For this review, take the finished solid that the model builds, in its own axes (mm). Round coordinates to 2 decimals unless told otherwise and drop trailing zeros. Write each loop counter-clockwise with the first axis right and the second up, starting at its lowest first coordinate (ties: lowest second). Pieces come first, ordered by that corner, then holes. Notation, with made-up numbers: (-31, 79) -> (-24, 79) arc R18 ccw to (-24, 83) -> close; hole circle Ø10 at (22, 85). An arc over 180 degrees is marked (long way). Write each question's results on one line, items separated by ' | '. Start each with the question number.
Item 1: Add section D-D (z = 2.2). State the section outline as (x, y) points.
Item 2: Add section B-B (y = 45.5). State the section outline as (x, z) points.
Item 3: Add section C-C (x = -1). State the section outline as (y, z) points, plus the area to 3 significant figures.
Item 4: To check wall thickness, follow line 1 along Z through (x, y) = (0, 5.25); line 2 along Y through (x, z) = (0, 1.4); line 3 along X through (y, z) = (53.75, 0). State the ranges of each line that lie inside material, in increasing order.
Item 5: Add section A-A (y = 9). State the section outline as (x, z) points.
Item 6: Clearance check with a flat-ended pin moving along its axis: pin 1 (1.8 mm diameter, centred on x = 0, z = 0, fed in from +Y). State where the tip first meets the part, or that it passes through.
from build123d import *

# Parameters (mm, degrees)
EXTRUDE_1_DEPTH     = 60
SKETCH_2_R          = 1.5
CUT_EXTRUDE_1_DEPTH = 10
SKETCH_3_R          = 1.5
CUT_EXTRUDE_2_DEPTH = 10


with BuildPart() as part:
    # Эскиз1 → Бобышка-Вытянуть1 (new body)
    with BuildSketch(Plane(origin=(0, 0, 0), x_dir=(1, 0, 0), z_dir=(0, 1, 0))):
        Polygon((-1.514417704, -2.79103428), (1.659897738, -2.707041343), (3.174315441, 0.083992937), (1.514417704, 2.79103428), (-1.659897738, 2.707041343), (-3.174315441, -0.083992937), align=None)
    extrude(amount=EXTRUDE_1_DEPTH)

    # Эскиз2 → Вырез-Вытянуть1 (cut)
    with BuildSketch(Plane(origin=(0, 60, 0), x_dir=(1, 0, 0), z_dir=(0, 1, 0))):
        Circle(SKETCH_2_R)
    extrude(amount=-CUT_EXTRUDE_1_DEPTH, mode=Mode.SUBTRACT)

    # Эскиз3 → Вырез-Вытянуть2 (cut)
    with BuildSketch(Plane.XZ):
        Circle(SKETCH_3_R)
    extrude(amount=-CUT_EXTRUDE_2_DEPTH, mode=Mode.SUBTRACT)


solid = part.part
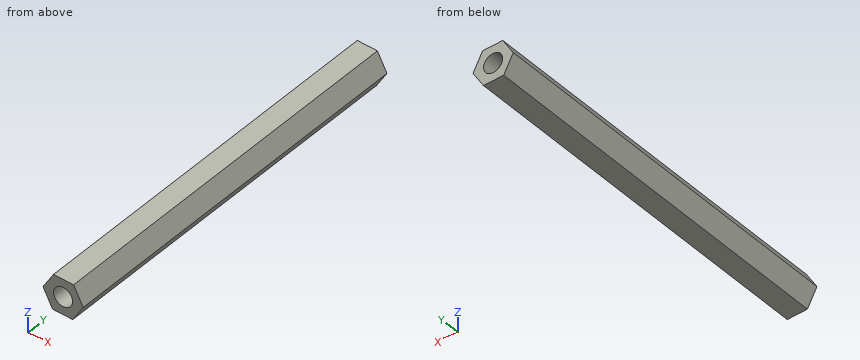
Responses:
1) outline: (-1.88, 0) -> (1.94, 0) -> (1.94, 60) -> (-1.88, 60) -> close
2) outline: (-3.17, 0.08) -> (-1.66, -2.71) -> (1.51, -2.79) -> (3.17, -0.08) -> (1.66, 2.71) -> (-1.51, 2.79) -> close
3) outline: (0, -2.72) -> (60, -2.72) -> (60, -1.12) -> (50, -1.12) -> (50, 1.12) -> (60, 1.12) -> (60, 2.78) -> (0, 2.78) -> (0, 1.12) -> (10, 1.12) -> (10, -1.12) -> (0, -1.12) -> close | area: 285 mm^2
4) line 1: z = -2.75 to -1.5, 1.5 to 2.75 | line 2: y = 10 to 50 | line 3: x = -3.13 to -1.5, 1.5 to 3.13
5) outline: (-3.17, 0.08) -> (-1.66, -2.71) -> (1.51, -2.79) -> (3.17, -0.08) -> (1.66, 2.71) -> (-1.51, 2.79) -> close; hole circle Ø3 at (0, 0)
6) pin 1: stops at y = 50
